The listing builds one solid part. Answer for the finished solid, in the listing's coordinates (mm). Give positions to 0.01 mm unless a question says otherwise; leave off trailing zeros. Order: outer loops, then holes, each group sorted by start corner. A loop starts at its lowest first (then second) coordinate and runs counter-clockwise, first axis right, second up. Notation, with made-up numbers: (43, 74) - (49, 74) arc R18 ccw to (49, 90) - close; hole circle Ø6 at (66, 65.5). An arc over 180 degrees is marked (long way). Answer as CSV lines item,"result". Start each with the question number.
1. Section A-A on z = 3 is taken. Give the vertices of the cut face in (x, y) (3 decimals).
2. A flat-ended cylindrical pin translates along its axis: pin 1 (1.9 mm diameter, centred on y = 773.5, z = 2, fed in from +X). Find the tip coordinate at first contact, or state that the pin passes through.
3. Section B-B on x = 57 is taken. Give the vertices of the cut face in (y, z), and give its area (3 significant figures).
4. Section C-C on x = 135.5 is taken. Give the vertices of the cut face in (y, z).
5. Consider line 1 along X through (y, z) = (666.75, 3.5) (3 decimals); line 2 along Y through (x, z) = (119.38, 4.5) (3 decimals); line 3 along X through (y, z) = (763, 2.75). Determine where each line is inside the solid, lowest interval first. Write a range as [from, to].
from build123d import *

# Parameters (mm, degrees)
BOSS_EXTRUDE1_DEPTH = 6.35
FILLET2_R           = 0.254
SKETCH2_R           = 3.175
CUT_EXTRUDE1_DEPTH  = 968.053696438


with BuildPart() as part:
    # Sketch1 → Boss-Extrude1 (new body)
    with BuildSketch(Plane.XY):
        Polygon((270.002, 0), (270.002, 757.893717478), (251.956545956, 757.893717478), (251.956545956, 783.293717478), (0, 928.76089711), (0, 0), align=None)
    extrude(amount=BOSS_EXTRUDE1_DEPTH)

    # Fillet2
    fillet2_edges = [part.edges().sort_by_distance(p)[0] for p in [
        (0, 0, 3.175),
        (0, 928.76089711, 3.175),
        (251.956545956, 783.293717478, 3.175),
        (251.956545956, 757.893717478, 3.175),
        (270.002, 757.893717478, 3.175),
    ]]
    fillet(fillet2_edges, radius=FILLET2_R)

    # Sketch2 → Cut-Extrude1 (cut, through all)
    with BuildSketch(Plane.XY.offset(6.35)):
        with Locations((119.38, 666.75)):
            Circle(SKETCH2_R)
    extrude(amount=-CUT_EXTRUDE1_DEPTH, mode=Mode.SUBTRACT)


solid = part.part
Checks:
1,outline,"(0, 0.254) arc R0.254 ccw to (0.254, 0) - (270.002, 0) - (270.002, 757.64) arc R0.254 ccw to (269.748, 757.894) - (252.211, 757.894) arc R0.254 cw to (251.957, 758.148) - (251.957, 783.147) arc R0.254 ccw to (251.83, 783.367) - (0.381, 928.541) arc R0.254 ccw to (0, 928.321) - close; hole circle Ø6.35 at (119.38, 666.75)"
2,pin 1,"stops at x = 251.96"
3,outline,"(0, 0) - (895.85, 0) - (895.85, 6.35) - (0, 6.35) - close"
3,area,"5,690 mm²"
4,outline,"(0, 0) - (850.53, 0) - (850.53, 6.35) - (0, 6.35) - close"
5,line 1,"x = [0, 116.205], [122.555, 270.002]"
5,line 2,"y = [0, 663.575], [669.925, 859.837]"
5,line 3,"x = [0, 251.96]"
